Check sheet for the drawn part. Datum: minimum x, y, z corner. Units: mm. A direction names the side the tool comes from. Give positions to 0.01 mm unless a question says otherwise; leave off trailing zeros. Order: outer loops, then holes, each group sorted by start corner. A loop starts at its lowest first (then second) coordinate and runs counter-clockwise, first axis right, second up. Notation, with made-up numbers: M 71,44 L 121,44 A12 cw 121,64 Z; hole C 86.5,34.5 d3. An arc over 180 degrees is marked long. Answer in a Markdown table with one row per item. Add a question column.
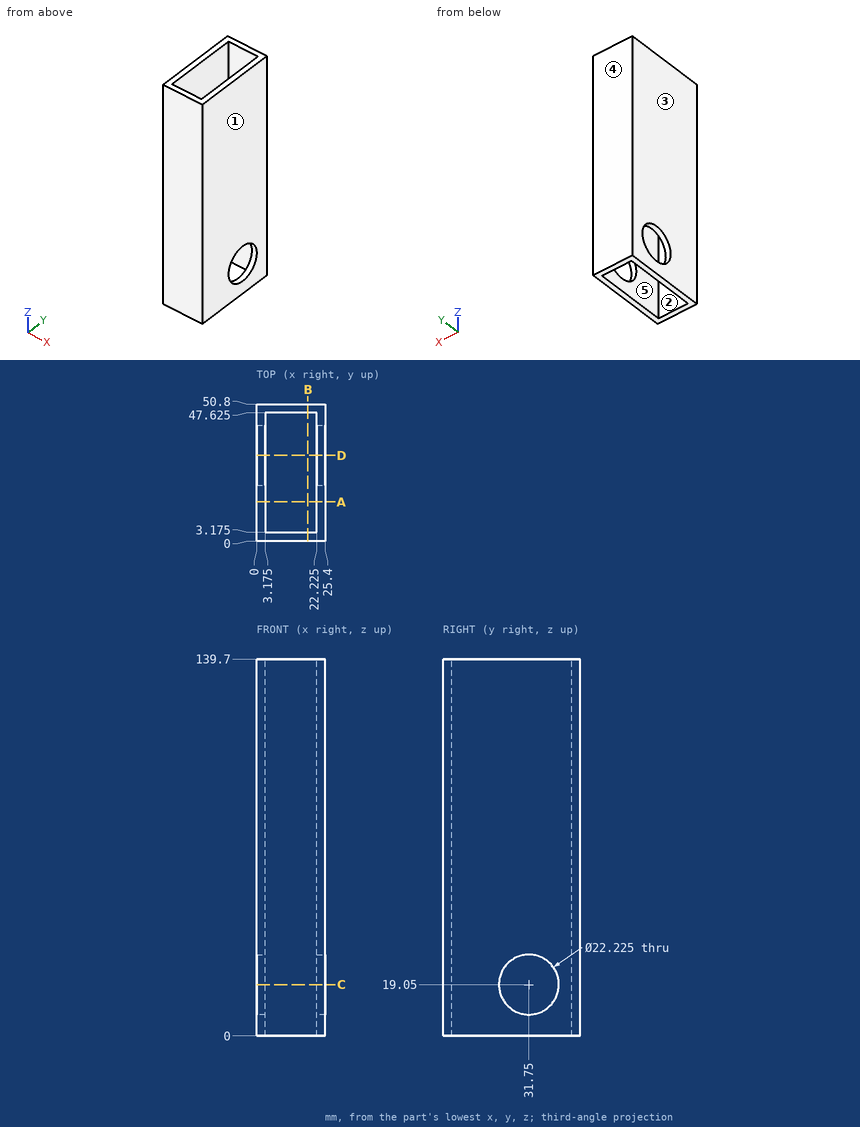
Q1. Cross-section at A-A (y = 14.5). Record the boundary of the cut face in (x, z) (3 decimals).
Q2. Cross-section at C-C (z = 19.05). Record the boundary of the cut face in (x, y) (1 decimal), and give its area (3 significant figures).
Q3. Tool access check on the marked faces 4 and 5. Record the directions out of +Z, -Z, +X, -X, +Y, -Y that give a thin tool (end or side, any length) a straight path to the whole face; none if there is none.
Q4. Cross-section at B-B (x = 19). Record the boundary of the cut face in (y, z) (3 decimals), and give its area (3 significant figures).
Q5. Draft check along X on the marked faces 1, 2 and 3. Enter one of: pulls with the +X half, pulls with the -X half, needs draft (parallel to the pull), parting line crosses it, or undercut.
Q6. Thickness scan on probe 1 along Y at (x, z) = (7, 77) (3 decimals); probe 2 along X at (y, z) = (26.5, 89.5) (3 decimals); probe 3 along Y at (x, z) = (0.7, 19.05). Record the ranges inside material, lowest first.
Q7. Cross-section at D-D (y = 31.75). Record the boundary of the cut face in (x, z) (1 decimal).
Values follow:
| question | item | result |
|---|---|---|
| 1 | outline | M 0,0 L 3.175,0 L 3.175,139.7 L 0,139.7 Z; M 22.225,0 L 25.4,0 L 25.4,139.7 L 22.225,139.7 Z |
| 2 | outline | M 0,0 L 25.4,0 L 25.4,20.6 L 22.2,20.6 L 22.2,3.2 L 3.2,3.2 L 3.2,20.6 L 0,20.6 Z; M 0,42.9 L 3.2,42.9 L 3.2,47.6 L 22.2,47.6 L 22.2,42.9 L 25.4,42.9 L 25.4,50.8 L 0,50.8 Z |
| 2 | area | 302 mm² |
| 3 | face 4 | +Z, -Z, +X, -X, +Y |
| 3 | face 5 | +Z, -Z |
| 4 | outline | M 0,0 L 3.175,0 L 3.175,139.7 L 0,139.7 Z; M 47.625,0 L 50.8,0 L 50.8,139.7 L 47.625,139.7 Z |
| 4 | area | 887 mm² |
| 5 | face 1 | pulls with the +X half |
| 5 | face 2 | undercut |
| 5 | face 3 | pulls with the -X half |
| 6 | probe 1 | 0 to 3.175, 47.625 to 50.8 |
| 6 | probe 2 | 0 to 3.175, 22.225 to 25.4 |
| 6 | probe 3 | 0 to 20.64, 42.86 to 50.8 |
| 7 | outline | M 0,0 L 3.2,0 L 3.2,7.9 L 0,7.9 Z; M 0,30.2 L 3.2,30.2 L 3.2,139.7 L 0,139.7 Z; M 22.2,0 L 25.4,0 L 25.4,7.9 L 22.2,7.9 Z; M 22.2,30.2 L 25.4,30.2 L 25.4,139.7 L 22.2,139.7 Z |
